Could you check a few things on this model? Use its own coordinates, in mm. A direction names the side the tool comes from. Round coordinates to 2 decimals unless told otherwise and drop trailing zeros. Write each loop counter-clockwise with the first axis right and the second up, starting at its lowest first coordinate (ties: lowest second). Pieces come first, ordered by that corner, then holes. Notation, with made-up numbers: (-11, 31.25) - (42, 31.25) arc R20 ccw to (42, 54.25) - close; hole circle Ø2 at (67, 34.25). An arc over 180 degrees is marked (long way). Put each result on its own line as item: value.
from build123d import *

# Parameters (mm, degrees)
SKETCH2_W               = 20.32
SKETCH2_H               = 7.62
SKETCH2_R               = 1.905
BOSS_EXTRUDE1_DEPTH     = 12.7
BOSS_EXTRUDE1_2_DEPTH   = 12.7
SKETCH4_W               = 7.62
SKETCH4_H               = 55.88
BOSS_EXTRUDE2_DEPTH     = 28.702
SKETCH5_W               = 27.94
SKETCH5_H               = 55.88
BOSS_EXTRUDE3_DEPTH     = 7.62
SKETCH6_R               = 10.922
BOSS_EXTRUDE6_DEPTH     = 55.88
SKETCH7_R               = 4.7625
CUT_EXTRUDE1_DEPTH      = 1
CUT_EXTRUDE1_DEPTH_BACK = 28.94
SKETCH8_W               = 27.94
SKETCH8_H               = 55.88
CUT_EXTRUDE2_DEPTH      = 29.702
CUT_EXTRUDE3_DEPTH      = 36.83
BOSS_EXTRUDE7_DEPTH     = 19.05


with BuildPart() as part:
    # Sketch2 → Boss-Extrude1 (new body)
    with BuildSketch(Plane.XY):
        with Locations((0, 24.13)):
            Rectangle(SKETCH2_W, SKETCH2_H)
        with Locations((4.699, 24.13)):
            Circle(SKETCH2_R, mode=Mode.SUBTRACT)
        with Locations((-4.699, 24.13)):
            Circle(SKETCH2_R, mode=Mode.SUBTRACT)
    extrude(amount=BOSS_EXTRUDE1_DEPTH)



with BuildPart() as body_2:
    # Sketch2 → Boss-Extrude1 2 (new body)
    with BuildSketch(Plane.XY):
        with Locations((0, -24.13)):
            Rectangle(SKETCH2_W, SKETCH2_H)
        with Locations((-4.699, -24.13)):
            Circle(SKETCH2_R, mode=Mode.SUBTRACT)
        with Locations((4.699, -24.13)):
            Circle(SKETCH2_R, mode=Mode.SUBTRACT)
    extrude(amount=BOSS_EXTRUDE1_2_DEPTH)


with BuildPart() as part_1:
    add(part.part)

    add(body_2.part)  # Boss-Extrude2 merges body 2
    # Sketch4 → Boss-Extrude2 (add)
    with BuildSketch(Plane.XY.offset(12.7)):
        with Locations((-13.97, 0)):
            Rectangle(SKETCH4_W, SKETCH4_H)
    extrude(amount=-BOSS_EXTRUDE2_DEPTH)

    # Sketch5 → Boss-Extrude3 (add)
    with BuildSketch(Plane(origin=(0, 0, -16.002), x_dir=(-1, 0, 0), z_dir=(0, 0, -1))):
        with Locations((3.81, 0)):
            Rectangle(SKETCH5_W, SKETCH5_H)
    extrude(amount=BOSS_EXTRUDE3_DEPTH)

    # Sketch6 → Boss-Extrude6 (add)
    with BuildSketch(Plane(origin=(0, 27.94, 0), x_dir=(1, 0, 0), z_dir=(0, 1, 0))):
        with BuildLine():
            Line((4.900385525, 23.622), (10.16, 23.622))
            Line((10.16, 23.622), (10.16, 34.544))
            ThreePointArc((10.16, 34.544), (-3.81, 48.514), (-17.78, 34.544))
            Line((-17.78, 34.544), (-17.78, 23.622))
            Line((-17.78, 23.622), (-12.520385525, 23.622))
            ThreePointArc((-12.520385525, 23.622), (-3.81, 20.574), (4.900385525, 23.622))
        make_face()
        with Locations((-3.81, 34.544)):
            Circle(SKETCH6_R, mode=Mode.SUBTRACT)
    extrude(amount=-BOSS_EXTRUDE6_DEPTH)

    # Sketch7 → Cut-Extrude1 (cut, two sides)
    with BuildSketch(Plane(origin=(10.16, 0, 0), x_dir=(0, 0, -1), z_dir=(1, 0, 0))) as cut_extrude1_sk:
        with Locations((34.544, 18.415)):
            Circle(SKETCH7_R)
    extrude(amount=CUT_EXTRUDE1_DEPTH, mode=Mode.SUBTRACT)
    extrude(cut_extrude1_sk.sketch, amount=-CUT_EXTRUDE1_DEPTH_BACK, mode=Mode.SUBTRACT)

    # Sketch8 → Cut-Extrude2 (cut, through all)
    with BuildSketch(Plane.XY.offset(-16.002)):
        with Locations((-3.81, 0)):
            Rectangle(SKETCH8_W, SKETCH8_H)
    extrude(amount=CUT_EXTRUDE2_DEPTH, mode=Mode.SUBTRACT)

    # Sketch9 → Cut-Extrude3 (cut)
    with BuildSketch(Plane(origin=(0, -27.94, 0), x_dir=(-1, 0, 0), z_dir=(0, -1, 0))):
        with BuildLine():
            Line((-10.16, 16.002), (17.78, 16.002))
            Line((17.78, 16.002), (17.78, 34.544))
            ThreePointArc((17.78, 34.544), (3.81, 48.514), (-10.16, 34.544))
            Line((-10.16, 34.544), (-10.16, 16.002))
        make_face()
    extrude(amount=-CUT_EXTRUDE3_DEPTH, mode=Mode.SUBTRACT)

    # Sketch10 → Boss-Extrude7 (add)
    with BuildSketch(Plane(origin=(0, 27.94, 0), x_dir=(1, 0, 0), z_dir=(0, 1, 0))):
        Polygon((-9.017, -39.878), (-9.017, -34.925), (-14.097, -34.925), (-14.097, -29.591), (6.477, -29.591), (6.477, -34.925), (1.397, -34.925), (1.397, -39.878), (10.16, -39.878), (10.16, 16.002), (-17.78, 16.002), (-17.78, -39.878), align=None)
    extrude(amount=-BOSS_EXTRUDE7_DEPTH)


solid = part_1.part
(1) I'm going to push flat-ended pins straight in: pin 1 (2 mm diameter, centred on y = 11.5, z = -36.5, fed in from +X); pin 2 (5.5 mm diameter, centred on x = -11.5, y = 20.5, fed in from -Z); pin 3 (1.5 mm diameter, centred on x = 3, y = 17.5, fed in from -Z). Where does each tip first touch, or does it pass through?
Values found:
pin 1: stops at x = 10.13
pin 2: stops at z = -47.61
pin 3: stops at z = -47.13
(2) Imagine slicing it at B-B, the plane y = 21. List the corners of the cut face in (x, z) for me (3 decimals), then the cut area to 3 significant figures.
Values found:
outline: (-17.78, -30.544) - (-13.973, -30.544) arc R10.922 cw to (6.353, -30.544) - (10.16, -30.544) - (10.16, 39.878) - (1.397, 39.878) - (1.397, 34.925) - (6.477, 34.925) - (6.477, 29.591) - (-14.097, 29.591) - (-14.097, 34.925) - (-9.017, 34.925) - (-9.017, 39.878) - (-17.78, 39.878) - close; (-17.195, -38.544) arc R13.97 ccw to (9.575, -38.544) - (6.353, -38.544) arc R10.922 cw to (-13.973, -38.544) - close
area: 1,800 mm^2
(3) Imagine slicing it at D-D, the plane x = 4.5. List the corners of the cut face in (y, z) for me (3 decimals).
Values found:
outline: (8.89, -45.774) - (27.94, -45.774) - (27.94, -41.632) - (8.89, -41.632) - close; (8.89, -27.456) - (27.94, -27.456) - (27.94, 29.591) - (8.89, 29.591) - close; (8.89, 34.925) - (27.94, 34.925) - (27.94, 39.878) - (8.89, 39.878) - close
(4) Please list where these lines run through material, in increasing order: probe 1 along Z at (x, y) = (-3.81, 15.5); probe 2 along Z at (x, y) = (-11.75, 24.25) (3 decimals); probe 3 along X at (y, z) = (26.25, 36.5). Write a range as from..to.
Values found:
probe 1: z = -48.51..-45.47, -23.62..29.59
probe 2: z = -46.038..-42.044, -27.044..29.591, 34.925..39.878
probe 3: x = -17.78..-9.02, 1.4..10.16
(5) Imagine slicing it at A-A, the plane x = -3.81. List the corners of the cut face in (y, z) for me.
Values found:
outline: (8.89, -48.51) - (27.94, -48.51) - (27.94, -45.47) - (8.89, -45.47) - close; (8.89, -23.62) - (27.94, -23.62) - (27.94, 29.59) - (8.89, 29.59) - close
(6) If we mould it in two halves opening along X, with no side actions, what happens to faces 1 (the face through (-13, 19, 39.878)), 2 (the face through (-17.78, 19, 2)), 3 (the face through (4, 19, 34.925))? For each: pulls with the +X half, pulls with the -X half, needs draft (parallel to the pull), parting line crosses it, or undercut.
Values found:
face 1: needs draft
face 2: pulls with the -X half
face 3: undercut
(7) Imagine slicing it at C-C, the plane z = -27. List the corners of the cut face in (x, y) for me, then the cut area to 3 significant figures.
Values found:
outline: (-17.78, 8.89) - (-11.71, 8.89) - (-11.71, 27.94) - (-17.78, 27.94) - close; (4.09, 8.89) - (10.16, 8.89) - (10.16, 27.94) - (4.09, 27.94) - close
area: 231 mm^2
(8) For faces 4 (the face through (1.397, 19, 37)), 5 (the face through (-14.097, 19, 32)), 6 (the face through (-3.5, 18.55, -48.51)), which set-ups out of +Z, -Z, +X, -X, +Y, -Y let a thin tool reach every point of the face, with its end or its side?
Values found:
face 4: +Z, +Y, -Y
face 5: +Y, -Y
face 6: -Z, +Y, -Y
